Read the model definition and answer for the solid it produces. Units are mm, in the model's axes. Give positions to 0.01 mm unless a question says otherwise; leave off trailing zeros. Order: outer loops, then holes, each group sorted by start corner. A loop starts at its lowest first (then second) coordinate and runs counter-clockwise, first axis right, second up. Notation, with made-up numbers: M 2.25,7.25 L 34.25,7.25 A21 ccw 34.25,11.25 Z; hole C 80.25,9.25 d3. An arc over 180 degrees is marked long. One line per item, written item: value.
from build123d import *

# Parameters (mm, degrees)
SKETCH2_W           = 203.2
SKETCH2_H           = 152.4
BOSS_EXTRUDE1_DEPTH = 12.7
SKETCH3_R           = 6.985
CUT_EXTRUDE1_DEPTH  = 128.633420388


with BuildPart() as part:
    # Sketch2 → Boss-Extrude1 (new body)
    with BuildSketch(Plane.XY):
        Rectangle(SKETCH2_W, SKETCH2_H)
    extrude(amount=BOSS_EXTRUDE1_DEPTH)

    # Sketch3 → Cut-Extrude1 (cut, through all)
    with BuildSketch(Plane(origin=(0, 0, 0), x_dir=(-1, 0, 0), z_dir=(0, 0, -1))):
        with Locations((53.975, 0)):
            Circle(SKETCH3_R)
        with Locations((85.725, 0)):
            Circle(SKETCH3_R)
        with Locations((53.975, -57.15)):
            Circle(SKETCH3_R)
        with Locations((-53.975, 0)):
            Circle(SKETCH3_R)
        with Locations(Location((53.975, 57.15, 0), (0, 0, 180))):
            Circle(SKETCH3_R)
        with Locations((-53.975, -57.15)):
            Circle(SKETCH3_R)
        with Locations((-85.725, 0)):
            Circle(SKETCH3_R)
        with Locations((-53.975, 57.15)):
            Circle(SKETCH3_R)
    extrude(amount=-CUT_EXTRUDE1_DEPTH, mode=Mode.SUBTRACT)


solid = part.part
1) Determine the mould class of faces 1 (the face through (50.22, -51.26, 6.26)), 2 (the face through (101.6, -1, 6)), 3 (the face through (-1, 1, 0)) for opening direction X: +X half, -X half, draft (parallel to the pull), parting line (faces both ways), or undercut.
Reported:
face 1: undercut
face 2: +X half
face 3: draft
2) Find section A-A, the plane y = -57.15. Write down the section's boundary in (x, z).
Reported:
outline: M -101.6,0 L -60.96,0 L -60.96,12.7 L -101.6,12.7 Z; M -46.99,0 L 46.99,0 L 46.99,12.7 L -46.99,12.7 Z; M 60.96,0 L 101.6,0 L 101.6,12.7 L 60.96,12.7 Z
3) Find section C-C, the plane x = 83.5. Write down the section's boundary in (y, z).
Reported:
outline: M -76.2,0 L -6.62,0 L -6.62,12.7 L -76.2,12.7 Z; M 6.62,0 L 76.2,0 L 76.2,12.7 L 6.62,12.7 Z
4) Consider probe 1 along Y at (x, z) = (-88.5, 9); probe 2 along Y at (x, z) = (88, 7.75). Determine where each line is inside the solid, lowest interval first.
Reported:
probe 1: y = -76.2 to -6.41, 6.41 to 76.2
probe 2: y = -76.2 to -6.6, 6.6 to 76.2
5) Find section D-D, the plane y = 0. Write down the section's boundary in (x, z).
Reported:
outline: M -101.6,0 L -92.71,0 L -92.71,12.7 L -101.6,12.7 Z; M -78.74,0 L -60.96,0 L -60.96,12.7 L -78.74,12.7 Z; M -46.99,0 L 46.99,0 L 46.99,12.7 L -46.99,12.7 Z; M 60.96,0 L 78.74,0 L 78.74,12.7 L 60.96,12.7 Z; M 92.71,0 L 101.6,0 L 101.6,12.7 L 92.71,12.7 Z
6) Find section B-B, the plane z = 8.25. Count the separate pieces of the cut face and the enclosed holes in it, plus the area to 3 significant figures.
Reported:
separate pieces: 1
enclosed holes: 8
area: 29,700 mm^2
7) This flat-tipped pin is pushed along its axis until it touches: pin 1 Ø16 at (x, y) = (53.975, 0) entering from +Z. Where does it stop, or does it pass through?
Reported:
pin 1: stops at z = 12.7
